Here's the drawing with two shaded views (mm, measured from the low corner). I have some questions. Coordinates: 2 decimals unless noted, no trailing zeros. Write each loop counter-clockwise with the first axis right and the second up, starting at its lowest first coordinate (ties: lowest second). Pieces come first, ordered by that corner, then holes.
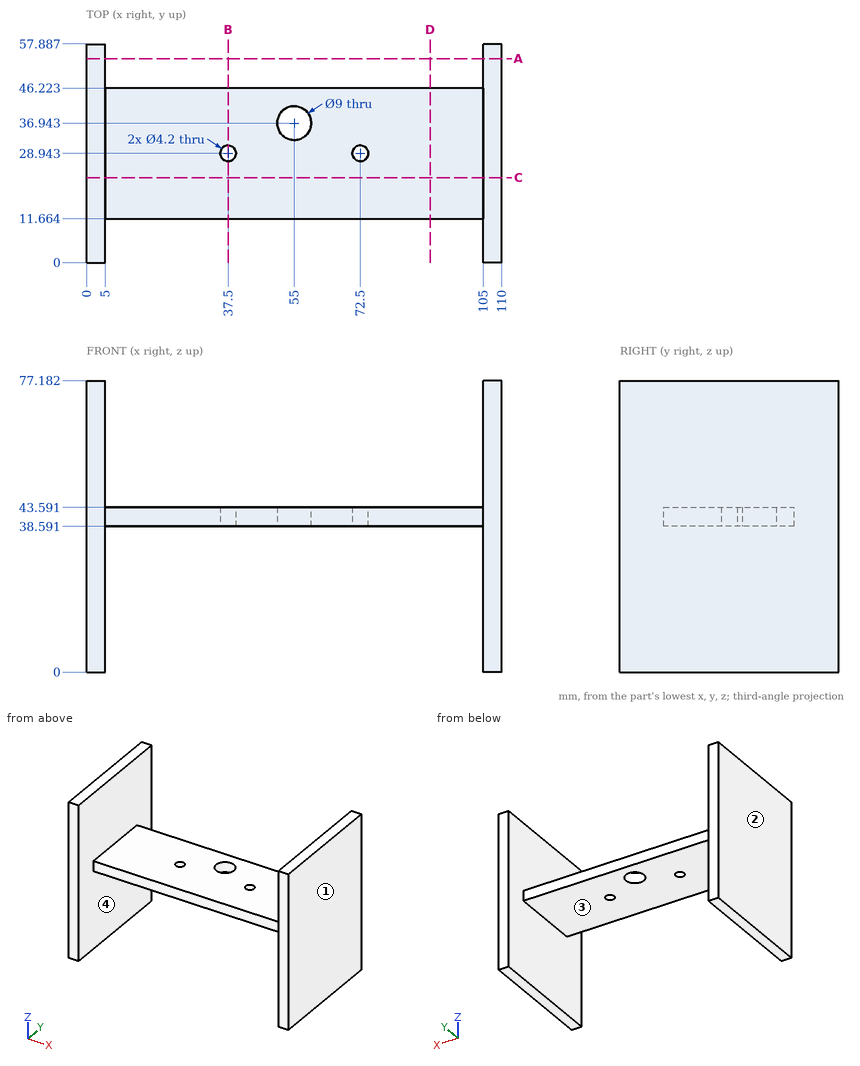
1. For pin 1 (2.5 mm diameter, centred on x = 31, z = 42, fed in from -Y); pin 2 (1 mm diameter, centred on x = 81.5, y = 17, fed in from -Z); pin 3 (7 mm diameter, centred on x = 55, y = 36.94, fed in from -Z); pin 4 (1.5 mm diameter, centred on x = 41.5, y = 37, fed in from +Z), each with a flat end and sliding along its axis, tell me the tip position at first contact or that it passes through.
Verdict:
pin 1: stops at y = 11.66
pin 2: stops at z = 38.59
pin 3: passes through
pin 4: stops at z = 43.59
2. I want a section at A-A on y = 54. Please give me the cut outline in (x, z), plus the area to 3 significant figures.
Verdict:
outline: (0, 0) - (5, 0) - (5, 77.18) - (0, 77.18) - close; (105, 0) - (110, 0) - (110, 77.18) - (105, 77.18) - close
area: 772 mm2
3. I want a section at B-B on x = 37.5. Please give me the cut outline in (y, z), plus the area to 3 significant figures.
Verdict:
outline: (11.66, 38.59) - (26.84, 38.59) - (26.84, 43.59) - (11.66, 43.59) - close; (31.04, 38.59) - (46.22, 38.59) - (46.22, 43.59) - (31.04, 43.59) - close
area: 152 mm2
4. I want a section at C-C on y = 22.5. Please give me the cut outline in (x, z).
Verdict:
outline: (0, 0) - (5, 0) - (5, 38.59) - (105, 38.59) - (105, 0) - (110, 0) - (110, 77.18) - (105, 77.18) - (105, 43.59) - (5, 43.59) - (5, 77.18) - (0, 77.18) - close
5. I want a section at D-D on x = 91. Please give me the cut outline in (y, z), plus the area to 3 significant figures.
Verdict:
outline: (11.66, 38.59) - (46.22, 38.59) - (46.22, 43.59) - (11.66, 43.59) - close
area: 173 mm2
6. Please list where these lines run through material, in increasing order: line 1 along X through (y, z) = (32.5, 48.5); line 2 along Y through (x, z) = (55, 40.95); line 3 along Z through (x, y) = (41.5, 13.5).
Verdict:
line 1: x = 0 to 5, 105 to 110
line 2: y = 11.66 to 32.44, 41.44 to 46.22
line 3: z = 38.59 to 43.59
7. If we mould it in two halves opening along X, with no side actions, what happens to the marked faces 1, 2, 3 and 4? For each: pulls with the +X half, pulls with the -X half, needs draft (parallel to the pull), parting line crosses it, or undercut.
Verdict:
face 1: pulls with the +X half
face 2: pulls with the -X half
face 3: undercut
face 4: undercut
